Part print with two shaded views. Sizes in mm from the minimum x, y, z corner. A direction names the side the tool comes from. Give positions to 0.01 mm unless a question says otherwise; leave off trailing zeros. Write each loop counter-clockwise with the first axis right and the second up, starting at its lowest first coordinate (ties: lowest second). Pieces come first, ordered by that corner, then holes. Notation, with made-up numbers: (56.25, 74) -> (81.25, 74) arc R35 ccw to (81.25, 110) -> close; hole circle Ø9 at (21, -19). An arc over 180 degrees is marked (long way). Answer as a JSON object with one key per item and string values.
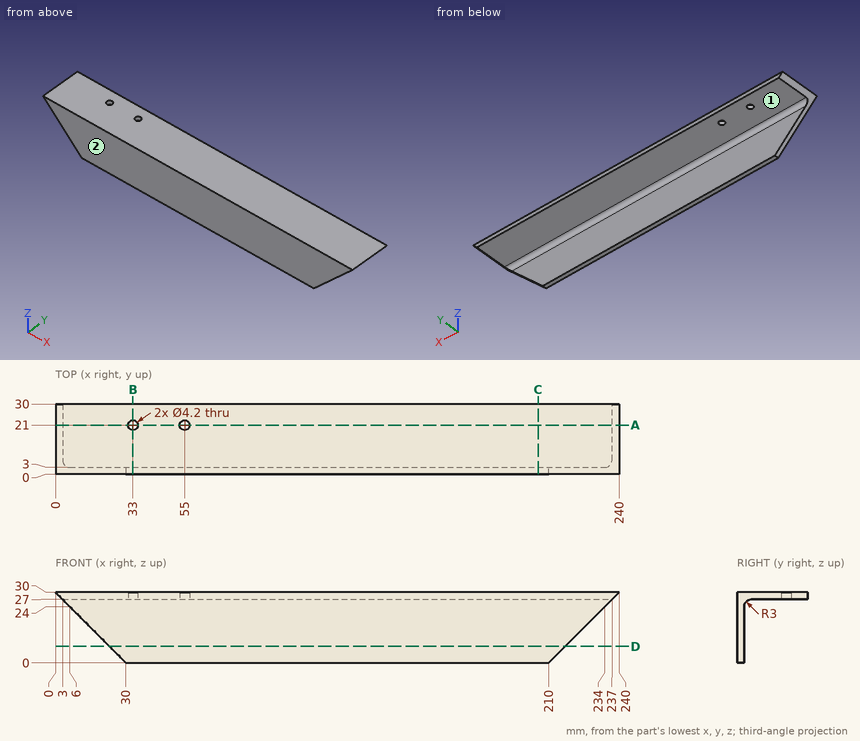
1) Pin check, flat tips, straight feed: pin 1 (2 mm diameter, centred on x = 162.5, z = 10.5, fed in from +Y); pin 2 (6 mm diameter, centred on x = 166, y = 24, fed in from -Z). Stop position of each tip, or through.
Model answer:
{"pin 1": "stops at y = 3", "pin 2": "stops at z = 27"}
2) 3-axis set-ups, long thin cutter, end or side, ignore diameter. For the marked faces 1 and 2: which of +Z, -Z, +X, -X, +Y, -Y reach the whole face in a straight line?
Model answer:
{"face 1": "-Z, +X, -X, +Y", "face 2": "+Z, -Z, +X, -X, -Y"}
3) Slice it at C-C (x = 205.5). List the corners of the cut face in (y, z).
Model answer:
{"outline": "(0, 0) -> (3, 0) -> (3, 24) arc R3 cw to (6, 27) -> (30, 27) -> (30, 30) -> (0, 30) -> close"}
4) Slice it at B-B (x = 33). List the corners of the cut face in (y, z), then the cut area to 3 significant figures.
Model answer:
{"outline": "(0, 0) -> (3, 0) -> (3, 24) arc R3 cw to (6, 27) -> (18.9, 27) -> (18.9, 30) -> (0, 30) -> close; (23.1, 27) -> (30, 27) -> (30, 30) -> (23.1, 30) -> close", "area": "160 mm2"}
5) Slice it at A-A (y = 21). List the corners of the cut face in (x, z), then the cut area to 3 significant figures.
Model answer:
{"outline": "(0, 30) -> (3, 27) -> (30.9, 27) -> (30.9, 30) -> close; (35.1, 27) -> (52.9, 27) -> (52.9, 30) -> (35.1, 30) -> close; (57.1, 27) -> (237, 27) -> (240, 30) -> (57.1, 30) -> close", "area": "686 mm2"}
6) Slice it at D-D (z = 7). List the corners of the cut face in (x, y).
Model answer:
{"outline": "(23, 0) -> (217, 0) -> (217, 3) -> (23, 3) -> close"}
7) Wall check: probe 1 along Y at (x, z) = (55, 28); probe 2 along Z at (x, y) = (144, 24.5); probe 3 along Y at (x, z) = (79, 19.5). Give the ranges that are in metal, low to high.
Model answer:
{"probe 1": "y = 0 to 18.9, 23.1 to 30", "probe 2": "z = 27 to 30", "probe 3": "y = 0 to 3"}
